Work out the finished part from the listing and answer in its coordinate system (mm). A direction names the side the tool comes from. Give positions to 0.01 mm unless a question says otherwise; leave off trailing zeros. Write each loop counter-clockwise with the first axis right and the second up, starting at its lowest first coordinate (ties: lowest second). Pieces come first, ordered by that corner, then holes. Notation, with made-up numbers: (19.5, -28) -> (25.5, -28) arc R27 ccw to (25.5, 6) -> close; hole circle Ø10 at (14, 80). An arc over 180 degrees is marked (long way). Use a Markdown table: item, result. Add a question column.
Q1. Section B-B, the plane y = 1.75 is taken. Give the vertices of the cut face in (x, z).
Q2. For a pull along X with two mould halves and no side action, classify faces 1 (the face through (0, 0, -0.7)), 2 (the face through (-8.2, 0, 4)), 3 (the face through (-7.5, 0, 4)) as pulls with the +X half, pulls with the -X half, needs draft (parallel to the pull), parting line crosses it, or undercut.
Q3. Section C-C, the plane x = -1 is taken. Give the vertices of the cut face in (y, z), plus the area to 3 significant figures.
Q4. Each of these flat-tipped pins is pushed along its axis until it touches: pin 1 Ø4 at (x, y) = (-13, 1) entering from -Z; pin 2 Ø2 at (y, z) = (-1, 1.5) entering from -X; pin 3 Ø5 at (y, z) = (2.5, 1.5) entering from +X; pin 4 Ø3 at (x, z) = (-10.5, 5) entering from +Y (3 decimals). Where does it stop, or does it pass through?
Q5. Consider line 1 (X direction, y = -3, z = 6.75); line 2 (Z direction, x = 0.5, y = 1.25); line 3 (X direction, y = -2.25, z = 0.25). Determine where each line is inside the solid, lowest interval first.
Q6. For faces 4 (the face through (12, 0, 8.3)), 5 (the face through (-14.215, -4.699, 8.645)), 6 (the face through (-12, 0, 8.3)), 7 (the face through (7.215, -0.07, 0.301)), 8 (the face through (12, 0, 9)), determine the directions among +Z, -Z, +X, -X, +Y, -Y from which every point of the face is accessible in a straight line to the end or side of a thin tool.
Q7. Section A-A, the plane z = 6.5 is taken. Give the vertices of the cut face in (x, y).
from build123d import *

# Parameters (mm, degrees)
SKETCH2_W                    = 15
SKETCH2_H                    = 10
BASE_FLANGE1_DEPTH           = 0.7
EDGE_FLANGE1_STRIP_W         = 4.8
EDGE_FLANGE1_STRIP_H         = 0.7
EDGE_FLANGE1_STRIP_CUT_DEPTH = 10
EDGE_FLANGE1_DEPTH           = 10
EDGE_FLANGE2_STRIP_W         = 4.8
EDGE_FLANGE2_STRIP_H         = 0.7
EDGE_FLANGE2_STRIP_CUT_DEPTH = 10
EDGE_FLANGE2_DEPTH           = 10
EDGE_FLANGE3_STRIP_W         = 4.8
EDGE_FLANGE3_STRIP_H         = 0.7
EDGE_FLANGE3_STRIP_CUT_DEPTH = 10
EDGE_FLANGE3_DEPTH           = 10
EDGE_FLANGE4_STRIP_W         = 4.8
EDGE_FLANGE4_STRIP_H         = 0.7
EDGE_FLANGE4_STRIP_CUT_DEPTH = 10
EDGE_FLANGE4_DEPTH           = 10
FILLET1_R                    = 1


# Sheet-metal steps are written as plain solids
with BuildPart() as part:
    # Sketch2 → Base-Flange1 (new body)
    with BuildSketch(Plane.XY):
        Rectangle(SKETCH2_W, SKETCH2_H)
    extrude(amount=-BASE_FLANGE1_DEPTH)

    # Edge-Flange1 strip (across the edge) → Edge-Flange1 strip cut (cut)
    with BuildSketch(Plane(origin=(-7.5, 5, 0), x_dir=(1, 0, 0), z_dir=(0, -1, 0))):
        with Locations((-1.4, -0.35)):
            Rectangle(EDGE_FLANGE1_STRIP_W, EDGE_FLANGE1_STRIP_H)
    extrude(amount=EDGE_FLANGE1_STRIP_CUT_DEPTH, mode=Mode.SUBTRACT)

    # Edge-Flange1 section (across the edge) → Edge-Flange1 (add)
    with BuildSketch(Plane(origin=(-7.5, 5, 0), x_dir=(1, 0, 0), z_dir=(0, -1, 0))):
        with BuildLine():
            Line((-0.7, 1), (-0.7, 8.3))
            Line((-0.7, 8.3), (0, 8.3))
            Line((0, 8.3), (0, 1))
            ThreePointArc((0, 1), (0.292893219, 0.292893219), (1, 0))
            Line((1, 0), (1, -0.7))
            ThreePointArc((1, -0.7), (-0.202081528, -0.202081528), (-0.7, 1))
        make_face()
    extrude(amount=EDGE_FLANGE1_DEPTH)

    # Edge-Flange2 strip (across the edge) → Edge-Flange2 strip cut (cut)
    with BuildSketch(Plane(origin=(7.5, -5, 0), x_dir=(-1, 0, 0), z_dir=(0, 1, 0))):
        with Locations((-1.4, -0.35)):
            Rectangle(EDGE_FLANGE2_STRIP_W, EDGE_FLANGE2_STRIP_H)
    extrude(amount=EDGE_FLANGE2_STRIP_CUT_DEPTH, mode=Mode.SUBTRACT)

    # Edge-Flange2 section (across the edge) → Edge-Flange2 (add)
    with BuildSketch(Plane(origin=(7.5, -5, 0), x_dir=(-1, 0, 0), z_dir=(0, 1, 0))):
        with BuildLine():
            Line((-0.7, 1), (-0.7, 8.3))
            Line((-0.7, 8.3), (0, 8.3))
            Line((0, 8.3), (0, 1))
            ThreePointArc((0, 1), (0.292893219, 0.292893219), (1, 0))
            Line((1, 0), (1, -0.7))
            ThreePointArc((1, -0.7), (-0.202081528, -0.202081528), (-0.7, 1))
        make_face()
    extrude(amount=EDGE_FLANGE2_DEPTH)

    # Edge-Flange3 strip (across the edge) → Edge-Flange3 strip cut (cut)
    with BuildSketch(Plane(origin=(8.2, 5, 8.3), x_dir=(0, 0, -1), z_dir=(0, -1, 0))):
        with Locations((-1.4, -0.35)):
            Rectangle(EDGE_FLANGE3_STRIP_W, EDGE_FLANGE3_STRIP_H)
    extrude(amount=EDGE_FLANGE3_STRIP_CUT_DEPTH, mode=Mode.SUBTRACT)

    # Edge-Flange3 section (across the edge) → Edge-Flange3 (add)
    with BuildSketch(Plane(origin=(8.2, 5, 8.3), x_dir=(0, 0, -1), z_dir=(0, -1, 0))):
        with BuildLine():
            Line((-0.7, 1), (-0.7, 6.3))
            Line((-0.7, 6.3), (0, 6.3))
            Line((0, 6.3), (0, 1))
            ThreePointArc((0, 1), (0.292893219, 0.292893219), (1, 0))
            Line((1, 0), (1, -0.7))
            ThreePointArc((1, -0.7), (-0.202081528, -0.202081528), (-0.7, 1))
        make_face()
    extrude(amount=EDGE_FLANGE3_DEPTH)

    # Edge-Flange4 strip (across the edge) → Edge-Flange4 strip cut (cut)
    with BuildSketch(Plane(origin=(-8.2, -5, 8.3), x_dir=(0, 0, -1), z_dir=(0, 1, 0))):
        with Locations((-1.4, -0.35)):
            Rectangle(EDGE_FLANGE4_STRIP_W, EDGE_FLANGE4_STRIP_H)
    extrude(amount=EDGE_FLANGE4_STRIP_CUT_DEPTH, mode=Mode.SUBTRACT)

    # Edge-Flange4 section (across the edge) → Edge-Flange4 (add)
    with BuildSketch(Plane(origin=(-8.2, -5, 8.3), x_dir=(0, 0, -1), z_dir=(0, 1, 0))):
        with BuildLine():
            Line((-0.7, 1), (-0.7, 6.3))
            Line((-0.7, 6.3), (0, 6.3))
            Line((0, 6.3), (0, 1))
            ThreePointArc((0, 1), (0.292893219, 0.292893219), (1, 0))
            Line((1, 0), (1, -0.7))
            ThreePointArc((1, -0.7), (-0.202081528, -0.202081528), (-0.7, 1))
        make_face()
    extrude(amount=EDGE_FLANGE4_DEPTH)

    # Fillet1
    fillet1_edges = [part.edges().sort_by_distance(p)[0] for p in [
        (14.5, -5, 8.65),
        (-14.5, -5, 8.65),
        (-14.5, 5, 8.65),
        (14.5, 5, 8.65),
    ]]
    fillet(fillet1_edges, radius=FILLET1_R)


solid = part.part
Result set:
| question | item | result |
|---|---|---|
| 1 | outline | (-14.5, 8.3) -> (-9.2, 8.3) arc R1 cw to (-8.2, 7.3) -> (-8.2, 1) arc R1.7 ccw to (-6.5, -0.7) -> (6.5, -0.7) arc R1.7 ccw to (8.2, 1) -> (8.2, 7.3) arc R1 cw to (9.2, 8.3) -> (14.5, 8.3) -> (14.5, 9) -> (9.2, 9) arc R1.7 ccw to (7.5, 7.3) -> (7.5, 1) arc R1 cw to (6.5, 0) -> (-6.5, 0) arc R1 cw to (-7.5, 1) -> (-7.5, 7.3) arc R1.7 ccw to (-9.2, 9) -> (-14.5, 9) -> close |
| 2 | face 1 | needs draft |
| 2 | face 2 | pulls with the -X half |
| 2 | face 3 | undercut |
| 3 | outline | (-5, -0.7) -> (5, -0.7) -> (5, 0) -> (-5, 0) -> close |
| 3 | area | 7.00 mm2 |
| 4 | pin 1 | stops at z = 8.3 |
| 4 | pin 2 | stops at x = -8.2 |
| 4 | pin 3 | stops at x = 8.2 |
| 4 | pin 4 | passes through |
| 5 | line 1 | x = -8.2 to -7.5, 7.5 to 8.2 |
| 5 | line 2 | z = -0.7 to 0 |
| 5 | line 3 | x = -8.03 to -7.16, 7.16 to 8.03 |
| 6 | face 4 | -Z, +X, +Y, -Y |
| 6 | face 5 | +Z, -Z, -X, -Y |
| 6 | face 6 | -Z, -X, +Y, -Y |
| 6 | face 7 | +Z, +Y, -Y |
| 6 | face 8 | +Z, +X, -X, +Y, -Y |
| 7 | outline | (-8.2, -5) -> (-7.5, -5) -> (-7.5, 5) -> (-8.2, 5) -> close; (7.5, -5) -> (8.2, -5) -> (8.2, 5) -> (7.5, 5) -> close |
